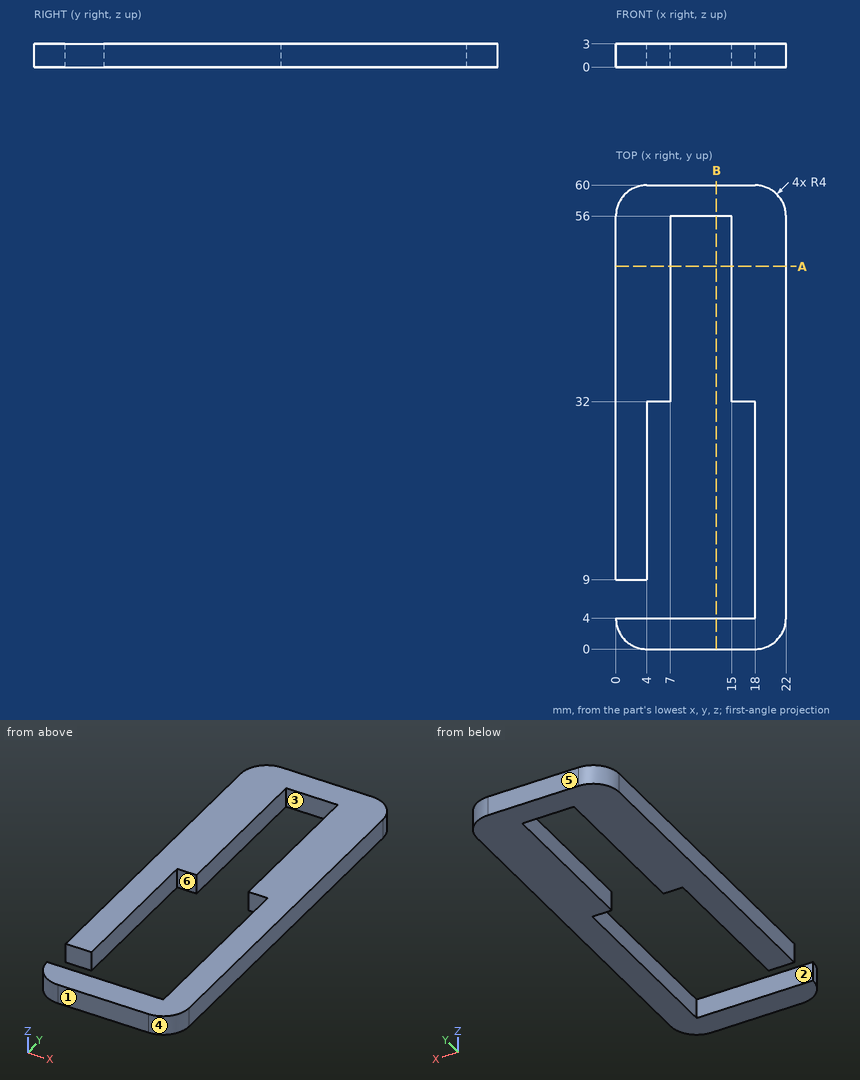
Here's the drawing with two shaded views (mm, measured from the low corner). I have some questions. A direction names the side the tool comes from. Give positions to 0.01 mm unless a question says otherwise; leave off trailing zeros. Order: outer loops, then holes, each group sorted by start corner. A loop starts at its lowest first (then second) coordinate and runs counter-clockwise, first axis right, second up. Notation, with made-up numbers: (52, 57.25) - (84, 57.25) arc R25 ccw to (84, 91.25) - close; hole circle Ø6 at (-40, 86). An arc over 180 degrees is marked (long way). Use a Markdown table: item, result. Add a question column.
Q1. If we mould it in two halves opening along Y, with no side actions, what happens to the marked faces 4, 5 and 6? For each: released by +Y, released by -Y, zero draft, split by the parting line, or undercut.
Q2. If we section it at B-B on x = 13: Write out the boundary of the cut face in (y, z), plus the area to 3 significant figures.
Q3. I'm going to push a flat-ended pin straight in: pin 1 (1 mm diameter, centred on x = 19.5, z = 1.5, fed in from -Y). Where does the tip first touch, or does it pass through?
Q4. If we section it at A-A on y = 49.5: Write out the boundary of the cut face in (x, z), plus the area to 3 significant figures.
Q5. Please list where these lines run through material, in increasing order: line 1 along X through (y, z) = (55.5, 2.6); line 2 along X through (y, z) = (26, 0.95); line 3 along Y through (x, z) = (17, 1.95).
Q6. On a 3-axis mill with a long thin cutter (end or side, diameter ignored), from which of +Z, -Z, +X, -X, +Y, -Y can I reach the whole of each face in a straight line? I mean the marked faces 1, 2 and 3. Say none if no direction works.
Answers follow:
| question | item | result |
|---|---|---|
| 1 | face 4 | released by -Y |
| 1 | face 5 | released by +Y |
| 1 | face 6 | undercut |
| 2 | outline | (0, 0) - (4, 0) - (4, 3) - (0, 3) - close; (56, 0) - (60, 0) - (60, 3) - (56, 3) - close |
| 2 | area | 24.0 mm^2 |
| 3 | pin 1 | stops at y = 0.13 |
| 4 | outline | (0, 0) - (7, 0) - (7, 3) - (0, 3) - close; (15, 0) - (22, 0) - (22, 3) - (15, 3) - close |
| 4 | area | 42.0 mm^2 |
| 5 | line 1 | x = 0 to 7, 15 to 22 |
| 5 | line 2 | x = 0 to 4, 18 to 22 |
| 5 | line 3 | y = 0 to 4, 32 to 60 |
| 6 | face 1 | +Z, -Z, +X, -X, -Y |
| 6 | face 2 | +Z, -Z, -X |
| 6 | face 3 | +Z, -Z |
